from build123d import *

# Parameters (mm, degrees)
SKIZZE1_W                       = 101.5
SKIZZE1_H                       = 26
AUFSATZ_LINEAR_AUSTRAGEN1_DEPTH = 3
VERRUNDUNG1_R                   = 10
SCHNITT_LINEAR_AUSTRAGEN2_REACH = 5
SKIZZE2_W                       = 3
SKIZZE2_H                       = 10


with BuildPart() as part:
    # Skizze1 → Aufsatz-Linear austragen1 (new body)
    with BuildSketch(Plane.XY):
        Polygon((0, 0), (59.172413793, 104), (198.476138787, 104), (139.303724994, 0), align=None)
        with Locations((82.738069394, 23)):
            Rectangle(SKIZZE1_W, SKIZZE1_H, mode=Mode.SUBTRACT)
        with Locations((115.738069394, 81)):
            Rectangle(SKIZZE1_W, SKIZZE1_H, mode=Mode.SUBTRACT)
    extrude(amount=AUFSATZ_LINEAR_AUSTRAGEN1_DEPTH)

    # Verrundung1
    verrundung1_edges = [part.edges().sort_by_distance(p)[0] for p in [
        (0, 0, 1.5),
        (59.172413793, 104, 1.5),
        (198.476138787, 104, 1.5),
        (139.303724994, 0, 1.5),
    ]]
    fillet(verrundung1_edges, radius=VERRUNDUNG1_R)

    # Skizze2 → Schnitt-Linear austragen2 (cut, up to next)
    with BuildSketch(Plane.XY.offset(3), mode=Mode.PRIVATE) as schnitt_linear_austragen2_sk1:
        with Locations((63.488069394, 81)):
            Rectangle(SKIZZE2_W, SKIZZE2_H)
    schnitt_linear_austragen2_tool1 = extrude(schnitt_linear_austragen2_sk1.sketch, amount=-SCHNITT_LINEAR_AUSTRAGEN2_REACH, mode=Mode.PRIVATE) & part.part
    add(schnitt_linear_austragen2_tool1.solids().sort_by_distance((63.488069, 81, 3))[0], mode=Mode.SUBTRACT)
    # Skizze2 → Schnitt-Linear austragen2 (cut, up to next)
    with BuildSketch(Plane.XY.offset(3), mode=Mode.PRIVATE) as schnitt_linear_austragen2_sk2:
        with Locations((167.988069394, 81)):
            Rectangle(SKIZZE2_W, SKIZZE2_H)
    schnitt_linear_austragen2_tool2 = extrude(schnitt_linear_austragen2_sk2.sketch, amount=-SCHNITT_LINEAR_AUSTRAGEN2_REACH, mode=Mode.PRIVATE) & part.part
    add(schnitt_linear_austragen2_tool2.solids().sort_by_distance((167.988069, 81, 3))[0], mode=Mode.SUBTRACT)
    # Skizze2 → Schnitt-Linear austragen2 (cut, up to next)
    with BuildSketch(Plane.XY.offset(3), mode=Mode.PRIVATE) as schnitt_linear_austragen2_sk3:
        with Locations((30.488069394, 23)):
            Rectangle(SKIZZE2_W, SKIZZE2_H)
    schnitt_linear_austragen2_tool3 = extrude(schnitt_linear_austragen2_sk3.sketch, amount=-SCHNITT_LINEAR_AUSTRAGEN2_REACH, mode=Mode.PRIVATE) & part.part
    add(schnitt_linear_austragen2_tool3.solids().sort_by_distance((30.488069, 23, 3))[0], mode=Mode.SUBTRACT)
    # Skizze2 → Schnitt-Linear austragen2 (cut, up to next)
    with BuildSketch(Plane.XY.offset(3), mode=Mode.PRIVATE) as schnitt_linear_austragen2_sk4:
        with Locations((134.988069394, 23)):
            Rectangle(SKIZZE2_W, SKIZZE2_H)
    schnitt_linear_austragen2_tool4 = extrude(schnitt_linear_austragen2_sk4.sketch, amount=-SCHNITT_LINEAR_AUSTRAGEN2_REACH, mode=Mode.PRIVATE) & part.part
    add(schnitt_linear_austragen2_tool4.solids().sort_by_distance((134.988069, 23, 3))[0], mode=Mode.SUBTRACT)


solid = part.part
Model file for the job. Use its own axes, mm. Round coordinates to 2 decimals unless told otherwise and drop trailing zeros. Loops run counter-clockwise (first coordinate to the right, second up) from the corner with the lowest first, then second, coordinate; pieces in that order, holes last. Notation, with made-up numbers: (-22.75, -35.5) -> (6.25, -35.5) arc R13 ccw to (6.25, -10.5) -> close; hole circle Ø2 at (-29.75, 15). An arc over 180 degrees is marked (long way). Answer as CSV lines item,"result". Start each with the question number.
1) Slice it at A-A (x = 103). List the corners of the cut face in (y, z), plus the area to 3 significant figures.
2) Slice it at C-C (x = 36). List the corners of the cut face in (y, z), plus the area to 3 significant figures.
3) Pin check, flat tips, straight feed: P1, Ø1.5, axis at y = 42.5, z = 1, coming from the -X side; P2, Ø1.5, axis at y = 32.5, z = 2, coming from the +X side; P3, Ø1.5, axis at x = 63.5, z = 1, coming from the +Y side; P4, Ø8, axis at x = 162, y = 26.5, coming from the +Z side. Stop position of each tip, or through.
4) Probe line 1 along Y through (x, z) = (107, 1.75); line 2 along Y through (x, z) = (144.5, 1.6); line 3 along Y through (x, z) = (64, 0.95). List the from-to ranges inside material, lowest first.
5) Slice it at D-D (y = 33.5). List the corners of the cut face in (x, z), plus the area to 3 significant figures.
6) Slice it at B-B (z = 1.85). State how many separate pieces and enclosed holes the cut face has, plus the area to 3 significant figures.
Filled in:
1,outline,"(0, 0) -> (10, 0) -> (10, 3) -> (0, 3) -> close; (36, 0) -> (68, 0) -> (68, 3) -> (36, 3) -> close; (94, 0) -> (104, 0) -> (104, 3) -> (94, 3) -> close"
1,area,"156 mm2"
2,outline,"(0, 0) -> (10, 0) -> (10, 3) -> (0, 3) -> close; (36, 0) -> (63.27, 0) -> (63.27, 3) -> (36, 3) -> close"
2,area,"112 mm2"
3,P1,"stops at x = 23.75"
3,P2,"stops at x = 158.22"
3,P3,"stops at y = 103.97"
3,P4,"passes through"
4,line 1,"y = 0 to 10, 36 to 68, 94 to 104"
4,line 2,"y = 9.13 to 68, 94 to 104"
4,line 3,"y = 0 to 10, 36 to 76, 86 to 103.95"
5,outline,"(19.06, 0) -> (31.99, 0) -> (31.99, 3) -> (19.06, 3) -> close; (133.49, 0) -> (158.36, 0) -> (158.36, 3) -> (133.49, 3) -> close"
5,area,"113 mm2"
6,separate pieces,"1"
6,enclosed holes,"2"
6,area,"8,940 mm2"
